Can you work these out from the model? Positions are in its coordinate system, mm. A direction names the side the tool comes from. Give positions to 0.01 mm unless a question says otherwise; leave off trailing zeros. Order: outer loops, then holes, each group sorted by start corner. A loop starts at its lowest first (then second) coordinate and runs counter-clockwise, first axis right, second up. Notation, with made-up numbers: M 89.25,82.5 L 99.25,82.5 A27 cw 99.25,113.5 Z; hole C 80,6 d3. An arc over 180 degrees is marked long. Use one line per item in the form item = value. Start each with the question number.
1. I want a section at B-B, the plane x = -27. List the corners of the cut face in (y, z) for me, and give its area (3 significant figures).
2. Will these pins go through, and if not, where does the flat tip stop? P1, Ø4, axis at x = -1.5, y = -9, coming from the +Z side; P2, Ø7.5, axis at x = -9.5, y = -1.5, coming from the -Z side; P3, Ø1.5, axis at y = -6, z = 9, coming from the -X side; P4, Ø3, axis at x = -14.5, z = 12, coming from the +Y side.
3. We'd pull the mould along Y, two halves only. Please class faces 4 (the face through (7.395, -1.498, -17.767)), 5 (the face through (7.4, -12.6, 12.71)), 6 (the face through (7.4, 17.82, -1.64)), 7 (the face through (7.4, 2.71, 15.26)): +Y half, -Y half, draft (parallel to the pull), parting line (faces both ways), or undercut.
4. I want a section at C-C, the plane x = -9. List the corners of the cut face in (y, z) for me, and give its area (3 significant figures).
5. For faces 1 (the face through (16.972, -3.755, 11.923)), 2 (the face through (7.395, -17.305, -4.555)), 3 (the face through (7.4, -12.57, -12.65)), which set-ups out of +Z, -Z, +X, -X, +Y, -Y let a thin tool reach every point of the face, with its end or its side?
6. I want a section at A-A, the plane z = 17. List the corners of the cut face in (x, y) for me, and give its area (3 significant figures).
7. I want a section at D-D, the plane x = 17.5. List the corners of the cut face in (y, z) for me, and give its area (3 significant figures).
8. I need wall thicknesses on L1, parallel to Y at x = 13.5, z = 17.5; L2, parallel to Y at x = 8.25, z = 0; L3, parallel to X at y = -10, z = 6. Which ranges of each line are inside material? Lowest first, please.
```python
from build123d import *

# Parameters (mm, degrees)
BASPROSKE_W         = 15
BASPROSKE_H         = 20
TOOTHCUT_DEPTH      = 33.015621187
TEETHCUTS_COUNT     = 18
TEETHCUTS_ANGLE     = 340
BORSKE_R            = 0.4
BORE_DEPTH          = 50.0000508
SKETCH1_R           = 12.5
BOSS_EXTRUDE1_DEPTH = 4
SKETCH1_3_R         = 10
BOSS_EXTRUDE2_DEPTH = 15
SKETCH2_W           = 1
SKETCH2_H           = 1
SKETCH3_R           = 14.5
BOSS_EXTRUDE3_DEPTH = 2
BOSS_EXTRUDE4_START = 17
SKETCH3_3_R         = 12.5
BOSS_EXTRUDE4_DEPTH = 17
BOSS_EXTRUDE5_START = 32
SKETCH3_4_R         = 10
BOSS_EXTRUDE5_DEPTH = 32
SKETCH4_W           = 1
SKETCH4_H           = 1
SKETCH5_OUTSIDE_W   = 58.744
SKETCH5_OUTSIDE_H   = 58.3
CUT_EXTRUDE1_DEPTH  = 15


with BuildPart() as part:
    # BasProSke → Base-Revolve (revolve)
    with BuildSketch(Plane(origin=(0, 0, 0), x_dir=(1, 0, 0), z_dir=(0, 1, 0)), mode=Mode.PRIVATE) as base_revolve_sk:
        with Locations((7.5, 10)):
            Rectangle(BASPROSKE_W, BASPROSKE_H)
    revolve(base_revolve_sk.sketch.rotate(Axis((-10, 0, 0), (1, 0, 0)), 180), axis=Axis((-10, 0, 0), (1, 0, 0)))

    # TooCutSke → ToothCut (cut, through all)
    with BuildSketch(Plane(origin=(0, 0, 0), x_dir=(0, 0, -1), z_dir=(1, 0, 0))):
        with BuildLine():
            ThreePointArc((1.007799284, 15.466199973), (0, 15.499), (-1.007799284, 15.466199973))
            ThreePointArc((-1.007799284, 15.466199973), (-1.630454606, 17.802374148), (-2.991345877, 19.800719558))
            ThreePointArc((-2.991345877, 19.800719558), (0, 20.0254), (2.991345877, 19.800719558))
            ThreePointArc((2.991345877, 19.800719558), (1.630454606, 17.802374148), (1.007799284, 15.466199973))
        make_face()
    toothcut = extrude(amount=TOOTHCUT_DEPTH, mode=Mode.SUBTRACT)

    # TeethCuts: ToothCut ×18 about axis
    teethcuts_axis = Axis((-10, 0, 0), (1, 0, 0))
    for i in range(1, TEETHCUTS_COUNT):
        add(toothcut.rotate(teethcuts_axis, i * TEETHCUTS_ANGLE / (TEETHCUTS_COUNT - 1)), mode=Mode.SUBTRACT)

    # BorSke → Bore (cut, symmetric)
    with BuildSketch(Plane(origin=(0, 0, 0), x_dir=(0, 0, -1), z_dir=(1, 0, 0))):
        with Locations(Location((0, 0, 0), (0, 0, 180))):
            Circle(BORSKE_R)
    extrude(amount=BORE_DEPTH, both=True, mode=Mode.SUBTRACT)

    # Sketch1 → Boss-Extrude1 (add)
    with BuildSketch(Plane(origin=(15, 0, 0), x_dir=(0, 0, -1), z_dir=(1, 0, 0))):
        with Locations(Location((0, 0, 0), (0, 0, 180))):
            Circle(SKETCH1_R)
    extrude(amount=BOSS_EXTRUDE1_DEPTH)

    # Sketch1<3> → Boss-Extrude2 (add)
    with BuildSketch(Plane(origin=(15, 0, 0), x_dir=(0, 0, -1), z_dir=(1, 0, 0))):
        Circle(SKETCH1_3_R)
    extrude(amount=BOSS_EXTRUDE2_DEPTH)

    # Sketch2 → Cut-Revolve1 (revolve, cut)
    with BuildSketch(Plane.XY, mode=Mode.PRIVATE) as cut_revolve1_sk:
        with Locations((19.5, 9.5)):
            Rectangle(SKETCH2_W, SKETCH2_H)
    revolve(cut_revolve1_sk.sketch.rotate(Axis((0, 0, 0), (1, 0, 0)), 90), axis=Axis((0, 0, 0), (1, 0, 0)), mode=Mode.SUBTRACT)

    # Sketch3 → Boss-Extrude3 (add)
    with BuildSketch(Plane.ZY):
        with Locations(Location((0, 0, 0), (0, 0, 180))):
            Circle(SKETCH3_R)
    extrude(amount=BOSS_EXTRUDE3_DEPTH)

    # Sketch3<3> → Boss-Extrude4 (add)
    with BuildSketch(Plane.ZY.offset(BOSS_EXTRUDE4_START)):
        Circle(SKETCH3_3_R)
    extrude(amount=-BOSS_EXTRUDE4_DEPTH)

    # Sketch3<4> → Boss-Extrude5 (add)
    with BuildSketch(Plane.ZY.offset(BOSS_EXTRUDE5_START)):
        Circle(SKETCH3_4_R)
    extrude(amount=-BOSS_EXTRUDE5_DEPTH)

    # Sketch4 → Cut-Revolve2 (revolve, cut)
    with BuildSketch(Plane.XY, mode=Mode.PRIVATE) as cut_revolve2_sk:
        with Locations((-21.5, 9.5)):
            Rectangle(SKETCH4_W, SKETCH4_H)
    revolve(cut_revolve2_sk.sketch.rotate(Axis((0, 0, 0), (-1, 0, 0)), 90), axis=Axis((0, 0, 0), (-1, 0, 0)), mode=Mode.SUBTRACT)

    # Sketch5 outside → Cut-Extrude1 (cut)
    with BuildSketch(Plane.ZY.offset(17)):
        Rectangle(SKETCH5_OUTSIDE_W, SKETCH5_OUTSIDE_H)
        with BuildLine():
            Line((-10, 7.5), (-10, -7.5))
            ThreePointArc((-10, -7.5), (0, -12.5), (10, -7.5))
            Line((10, -7.5), (10, 7.5))
            ThreePointArc((10, 7.5), (0, 12.5), (-10, 7.5))
        make_face(mode=Mode.SUBTRACT)
    extrude(amount=-CUT_EXTRUDE1_DEPTH, mode=Mode.SUBTRACT)


solid = part.part
```
Check result:
q1.outline = C 0,0 d20
q1.area = 314 mm2
q2.P1 = 14.61
q2.P2 = -10
q2.P3 = -17
q2.P4 = through
q3.face_4 = undercut
q3.face_5 = -Y half
q3.face_6 = +Y half
q3.face_7 = undercut
q4.outline = M -7.5,-10 L 7.5,-10 A12.5 ccw 7.5,10 L -7.5,10 A12.5 ccw Z
q4.area = 440 mm2
q5.face_1 = +X
q5.face_2 = +X, -X
q5.face_3 = +X, -X, -Y
q6.outline = M 0,-7.52 L 15,-7.52 L 15,-4.53 L 0,-4.53 Z; M 0,-1.65 L 15,-1.65 L 15,1.65 L 0,1.65 Z; M 0,4.53 L 15,4.53 L 15,7.52 L 0,7.52 Z
q6.area = 139 mm2
q7.outline = C 0,0 d25
q7.area = 491 mm2
q8.L1 = -7.5 to -4.88, -1.56 to 1.56, 4.88 to 7.5
q8.L2 = -15.5 to -0.4, 0.4 to 15.5
q8.L3 = -17 to 19
